Model file for the job. Use its own axes, mm. Round coordinates to 2 decimals unless told otherwise and drop trailing zeros. Loops run counter-clockwise (first coordinate to the right, second up) from the corner with the lowest first, then second, coordinate; pieces in that order, holes last. Notation, with made-up numbers: M -6,6.25 L 14,6.25 A18 ccw 14,27.25 Z; hole C 58,35.5 d1. An arc over 180 degrees is marked long. Use a Markdown table: item, result. Add a question column.
Q1. Pin check, flat tip, straight feed: pin 1 (2.5 mm diameter, centred on x = -199.5, y = 110.5, fed in from -Z). Stop position of the tip, or through.
Q2. Cut at B-B (x = -194). Give the cut face in (y, z).
Q3. Cut at A-A (y = 111). Give the cut face in (x, z).
Q4. Probe line 1 (Y direction, x = -196.75, z = -0.8); line 2 (Y direction, x = -201.75, z = -0.75); line 3 (X direction, y = 113, z = -0.5). List the from-to ranges inside material, lowest first. Write a range as from..to.
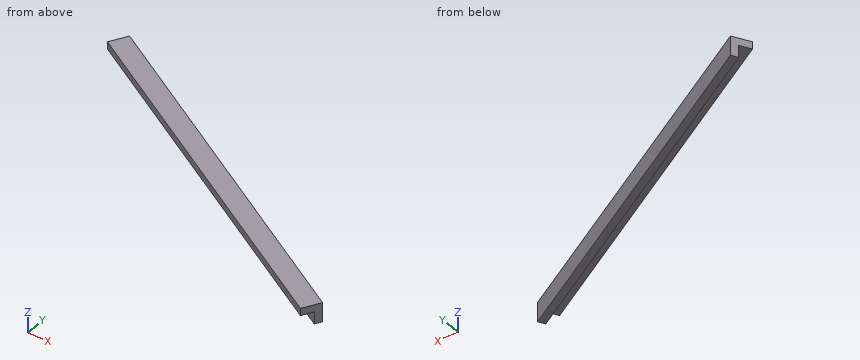
from build123d import *

# Parameters (mm, degrees)
BOX121_W               = 0.8
BOX121_H               = 16
BOX121_DEPTH           = 0.8
BOX122_W               = 0.8
BOX122_H               = 16
BOX122_DEPTH           = 0.8
CUT064_PLACEMENT_ANGLE = 61


with BuildPart() as cubo121:
    # Box121 → Box121 (new body)
    with BuildSketch(Plane.XY):
        with Locations((0.4, 8)):
            Rectangle(BOX121_W, BOX121_H)
    extrude(amount=BOX121_DEPTH)


with BuildPart() as obj1:
    # Box122 → Box122 (new body)
    with BuildSketch(Plane(origin=(0.3, 0, 0.3), x_dir=(1, 0, 0), z_dir=(0, 0, 1))):
        with Locations((0.4, 8)):
            Rectangle(BOX122_W, BOX122_H)
    extrude(amount=BOX122_DEPTH)

    # Cut064: cut Cubo121
    add(cubo121.part, mode=Mode.SUBTRACT)


with BuildPart() as obj1_1:
    # Cut064 placement: moved
    add(obj1.part.moved(Location((-191.4, 105.3, -1.45))).rotate(Axis((-191.4, 105.3, -1.45), (0, 0, 1)), CUT064_PLACEMENT_ANGLE))


solid = obj1_1.part
Checked values:
| question | item | result |
|---|---|---|
| 1 | pin 1 | stops at z = -1.15 |
| 2 | outline | M 107.08,-0.65 L 107.66,-0.65 L 107.66,-1.15 L 108,-1.15 L 108,-0.35 L 107.08,-0.35 Z |
| 3 | outline | M -201.06,-0.65 L -200.03,-0.65 L -200.03,-1.15 L -199.41,-1.15 L -199.41,-0.35 L -201.06,-0.35 Z |
| 4 | line 1 | y = 109.18..109.52 |
| 4 | line 2 | y = 111.95..112.29 |
| 4 | line 3 | x = -204.67..-203.02 |
